Work out the finished part from the listing and answer in its coordinate system (mm). Face numbers are marked on the shaded views. A direction names the side the tool comes from. Give positions to 0.01 mm unless a question says otherwise; leave off trailing zeros. Order: outer loops, then holes, each group sorted by start corner. A loop starts at its lowest first (then second) coordinate and runs counter-clockwise, first axis right, second up. Notation, with made-up numbers: (26.25, 30.25) - (60.25, 30.25) arc R3 ccw to (60.25, 35.25) - close; hole circle Ø8 at (63.25, 63). An arc over 180 degrees is marked (long way). Put each result on its own line as item: value.
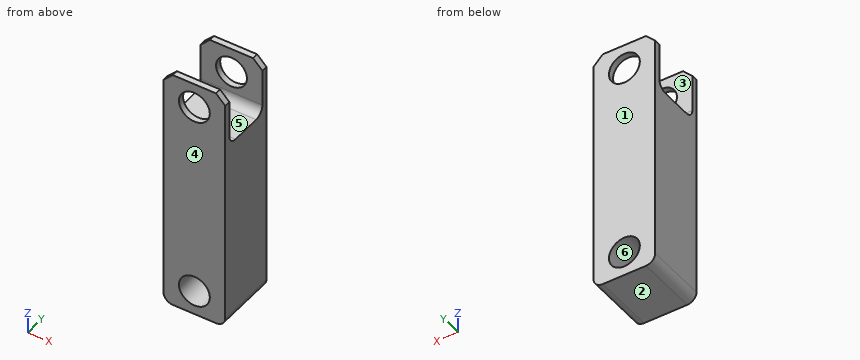
```python
from build123d import *

# Parameters (mm, degrees)
SKETCH1_W           = 20
SKETCH1_H           = 20
BOSS_EXTRUDE1_DEPTH = 80
SKETCH2_R           = 5
CUT_EXTRUDE1_DEPTH  = 80
SKETCH3_W           = 20
SKETCH3_H           = 16
CUT_EXTRUDE2_DEPTH  = 18
SKETCH4_R           = 5
CUT_EXTRUDE3_DEPTH  = 92
FILLET1_R           = 3
CHAMFER1_SIZE       = 3


with BuildPart() as part:
    # Sketch1 → Boss-Extrude1 (new body)
    with BuildSketch(Plane.XY):
        Rectangle(SKETCH1_W, SKETCH1_H)
    extrude(amount=BOSS_EXTRUDE1_DEPTH)

    # Sketch2 → Cut-Extrude1 (cut)
    with BuildSketch(Plane(origin=(0, 10, 0), x_dir=(1, 0, 0), z_dir=(0, 1, 0))):
        with Locations(Location((0, -8, 0), (0, 0, 270))):
            Circle(SKETCH2_R)
    extrude(amount=-CUT_EXTRUDE1_DEPTH, mode=Mode.SUBTRACT)

    # Sketch3 → Cut-Extrude2 (cut)
    with BuildSketch(Plane.XY.offset(80)):
        Rectangle(SKETCH3_W, SKETCH3_H)
    extrude(amount=-CUT_EXTRUDE2_DEPTH, mode=Mode.SUBTRACT)

    # Sketch4 → Cut-Extrude3 (cut)
    with BuildSketch(Plane.XZ.offset(10)):
        with Locations(Location((0, 72, 0), (0, 0, 270))):
            Circle(SKETCH4_R)
    extrude(amount=-CUT_EXTRUDE3_DEPTH, mode=Mode.SUBTRACT)

    # Fillet1
    fillet1_edges = [part.edges().sort_by_distance(p)[0] for p in [
        (0, 8, 62),
        (0, -8, 62),
        (-10, 0, 0),
        (10, 0, 0),
    ]]
    fillet(fillet1_edges, radius=FILLET1_R)

    # Chamfer1
    chamfer1_edges = [part.edges().sort_by_distance(p)[0] for p in [
        (-10, 9, 80),
        (10, 9, 80),
        (-10, -9, 80),
        (10, -9, 80),
    ]]
    chamfer(chamfer1_edges, length=CHAMFER1_SIZE)


solid = part.part
```
(1) Straight lines are drawn through the part: line 1 (X direction, y = -2.5, z = 8); line 2 (Y direction, x = 2.25, z = 77.5); line 3 (Z direction, x = -4, y = -4.75). For each, find the intervals that lie inside material, in ascending order.
Geometry check:
line 1: x = -10 to -5, 5 to 10
line 2: y = -10 to -8, 8 to 10
line 3: z = 0 to 5, 11 to 62
(2) Section C-C, the plane z = 72 is taken. Write down the section's boundary in (x, y), then the cut area to 3 significant figures.
Geometry check:
outline: (-10, -10) - (-5, -10) - (-5, -8) - (-10, -8) - close; (-10, 8) - (-5, 8) - (-5, 10) - (-10, 10) - close; (5, -10) - (10, -10) - (10, -8) - (5, -8) - close; (5, 8) - (10, 8) - (10, 10) - (5, 10) - close
area: 40.0 mm²
(3) A tool of negligible diameter and unlimited length cuts with its end or side. For the marked faces 5 and 6, from which of +Z, -Z, +X, -X, +Y, -Y can it reach the whole face along a straight path? Write none if from no direction.
Geometry check:
face 5: +Z, +X, -X
face 6: +Y, -Y
(4) Section D-D, the plane y = 6 is taken. Write down the section's boundary in (x, z), then the cut area to 3 significant figures.
Geometry check:
outline: (-10, 3) arc R3 ccw to (-7, 0) - (7, 0) arc R3 ccw to (10, 3) - (10, 62.17) - (-10, 62.17) - close; hole circle Ø10 at (0, 8)
area: 1,160 mm²
(5) Section A-A, the plane x = 3 is taken. Write down the section's boundary in (y, z).
Geometry check:
outline: (-10, 0) - (10, 0) - (10, 4) - (-10, 4) - close; (-10, 12) - (10, 12) - (10, 68) - (8, 68) - (8, 65) arc R3 cw to (5, 62) - (-5, 62) arc R3 cw to (-8, 65) - (-8, 68) - (-10, 68) - close; (-10, 76) - (-8, 76) - (-8, 80) - (-10, 80) - close; (8, 76) - (10, 76) - (10, 80) - (8, 80) - close
(6) Section B-B, the plane z = 8 is taken. Write down the section's boundary in (x, y).
Geometry check:
outline: (-10, -10) - (-5, -10) - (-5, 10) - (-10, 10) - close; (5, -10) - (10, -10) - (10, 10) - (5, 10) - close
(7) Determine the mould class of the marked faces 1, 2, 3 and 4 for opening direction Y: pulls with the +Y half, pulls with the -Y half, needs draft (parallel to the pull), parting line crosses it, or undercut.
Geometry check:
face 1: pulls with the +Y half
face 2: needs draft
face 3: undercut
face 4: pulls with the -Y half
(8) Given pin 1 (9 mm diameter, centred on x = 0, z = 72, fed in from +Y); pin 2 (8 mm diameter, centred on x = 1.5, y = 1.5, fed in from +Z), each flat-ended and moving along its own axis, determine where each tip first touches the part or whether it passes through.
Geometry check:
pin 1: passes through
pin 2: stops at z = 62.04
